Verification items for this drawing (mm, ordinates from the low corner). A direction names the side the tool comes from. Give positions to 0.01 mm unless a question says otherwise; leave off trailing zeros. Loops run counter-clockwise (first coordinate to the right, second up) from the corner with the lowest first, then second, coordinate; pieces in that order, holes last. Notation, with made-up numbers: M 46.5,22.25 L 73.5,22.25 A10 cw 73.5,30.25 Z; hole C 85.25,51 d10. An arc over 180 degrees is marked long. Answer in a Markdown table with one row per item.
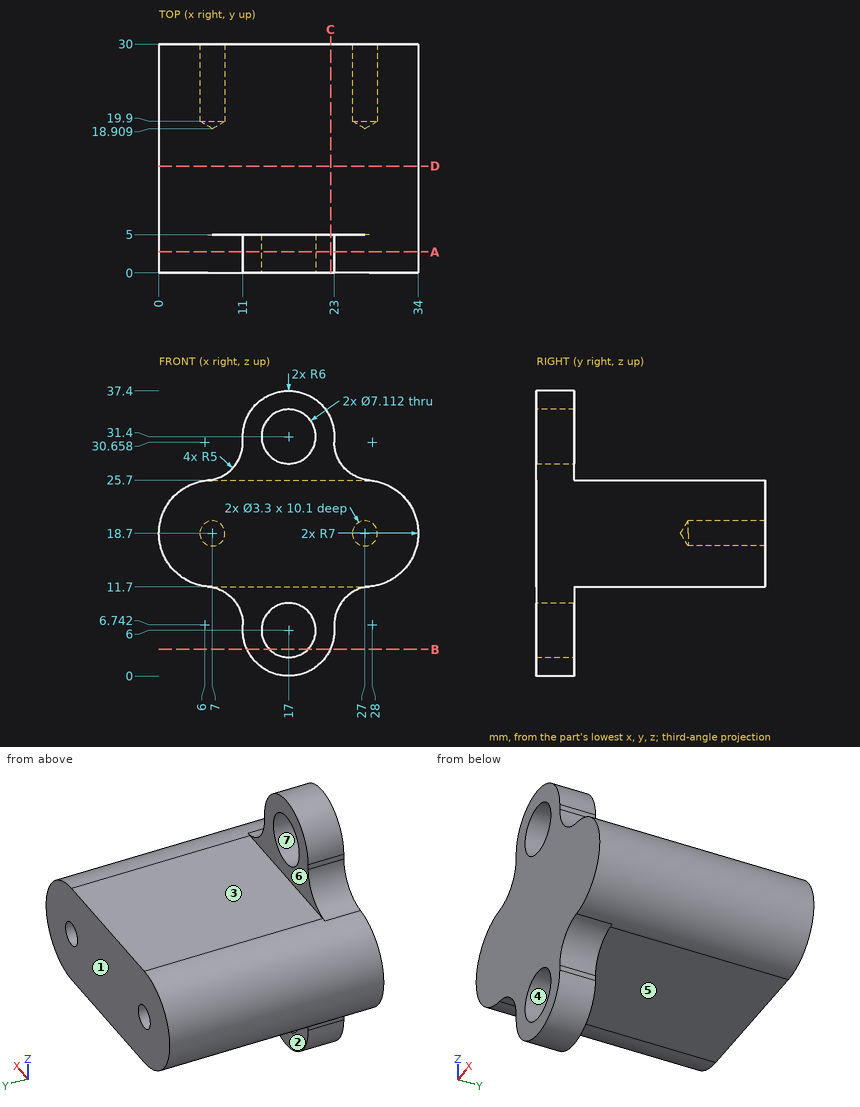
Item 1: Tool access check on the marked faces 1, 2 and 3. Record the directions out of +Z, -Z, +X, -X, +Y, -Y that give a thin tool (end or side, any length) a straight path to the whole face; none if there is none.
Reported:
| item | result |
|---|---|
| face 1 | +Z, -Z, +X, -X, +Y |
| face 2 | -Z, +X, -X, +Y |
| face 3 | +Z, +X, -X, +Y |
Item 2: Go/stop test with flat-tipped pins: pin 1 (4 mm diameter, centred on x = 8, y = 10.5, fed in from +Z); pin 2 (6 mm diameter, centred on x = 18, y = 17, fed in from -Z); pin 3 (0.6 mm diameter, centred on y = 3.5, z = 6.5, fed in from -X). Record where each tip stops, or that it passes through.
Reported:
| item | result |
|---|---|
| pin 1 | stops at z = 25.7 |
| pin 2 | stops at z = 11.7 |
| pin 3 | stops at x = 11 |
Item 3: Sectioned sample at B-B (z = 3.5). Record the cut outline in (x, y) (1 decimal).
Reported:
| item | result |
|---|---|
| outline | M 11.5,0 L 14.5,0 L 14.5,5 L 11.5,5 Z; M 19.5,0 L 22.5,0 L 22.5,5 L 19.5,5 Z |
Item 4: Sectioned sample at D-D (y = 14). Record the cut outline in (x, z), and give its area (3 significant figures).
Reported:
| item | result |
|---|---|
| outline | M 7,11.7 L 27,11.7 A7 ccw 27,25.7 L 7,25.7 A7 ccw Z |
| area | 434 mm^2 |
Item 5: Sectioned sample at A-A (y = 2.75). Record the cut outline in (x, z) (1 decimal), and give its area (3 significant figures).
Reported:
| item | result |
|---|---|
| outline | M 6.4,11.7 A5 cw 11,6.7 L 11,6 A6 ccw 23,6 L 23,6.7 A5 cw 27.6,11.7 A7 ccw 27.6,25.7 A5 cw 23,30.7 L 23,31.4 A6 ccw 11,31.4 L 11,30.7 A5 cw 6.4,25.7 A7 ccw Z; hole C 17,6 d7.1; hole C 17,31.4 d7.1 |
| area | 625 mm^2 |
Item 6: Sectioned sample at C-C (x = 22.5). Record the cut outline in (y, z), and give its area (3 significant figures).
Reported:
| item | result |
|---|---|
| outline | M 0,3.6 L 5,3.6 L 5,11.7 L 30,11.7 L 30,25.7 L 5,25.7 L 5,33.8 L 0,33.8 Z |
| area | 501 mm^2 |
Item 7: Scan lines: L1, parallel to X at y = 25.25, z = 18.7; L2, parallel to Y at x = 14, z = 34.5; L3, parallel to Z at x = 27, y = 27.75. Record each from-to range of solid material in increasing order. Write a range as [from, to].
Reported:
| item | result |
|---|---|
| L1 | x = [0, 5.35], [8.65, 25.35], [28.65, 34] |
| L2 | y = [0, 5] |
| L3 | z = [11.7, 17.05], [20.35, 25.7] |
Item 8: Release check for a two-part mould opening along Z. For the marked faces 4, 5, 6 and 7 record: released by +Z, released by -Z, zero draft, split by the parting line, or undercut.
Reported:
| item | result |
|---|---|
| face 4 | undercut |
| face 5 | released by -Z |
| face 6 | zero draft |
| face 7 | undercut |
